Geometry: final body of the model. Coordinates: model frame, mm. A direction names the side the tool comes from. Give positions to 0.01 mm unless a question says otherwise; leave off trailing zeros. Loops run counter-clockwise (first coordinate to the right, second up) from the corner with the lowest first, then second, coordinate; pieces in that order, holes last. Notation, with made-up numbers: (-8, 59) - (20, 59) arc R20 cw to (20, 76) - close; hole circle Ø1 at (29, 48). An arc over 180 degrees is marked (long way). Answer in a Markdown table with one row per item.
from build123d import *

# Parameters (mm, degrees)
SKETCH1_R           = 1.5
BOSS_EXTRUDE1_DEPTH = 38.15
SKETCH4_W           = 9.31
SKETCH4_H           = 38.15
CUT_EXTRUDE2_DEPTH  = 45


with BuildPart() as part:
    # Sketch1 → Boss-Extrude1 (new body)
    with BuildSketch(Plane(origin=(0, 0, 0), x_dir=(1, 0, 0), z_dir=(0, 1, 0))):
        with BuildLine():
            Line((-43.3, 25.002199903), (-19.589917361, 15.692199903))
            ThreePointArc((-19.589917361, 15.692199903), (25.1, 0), (-19.589917361, -15.692199903))
            Line((-19.589917361, -15.692199903), (-43.3, -25.002199903))
            ThreePointArc((-43.3, -25.002199903), (50, 0), (-43.3, 25.002199903))
        make_face()
        with Locations(Location((8, -35.55, 0), (0, 0, 270))):
            Circle(SKETCH1_R, mode=Mode.SUBTRACT)
        with Locations(Location((-8, -35.55, 0), (0, 0, 90))):
            Circle(SKETCH1_R, mode=Mode.SUBTRACT)
        with Locations(Location((8, 35.55, 0), (0, 0, 90))):
            Circle(SKETCH1_R, mode=Mode.SUBTRACT)
        with Locations(Location((-8, 35.55, 0), (0, 0, 270))):
            Circle(SKETCH1_R, mode=Mode.SUBTRACT)
        with Locations(Location((35.55, 8, 0), (0, 0, 270))):
            Circle(SKETCH1_R, mode=Mode.SUBTRACT)
        with Locations(Location((35.55, -8, 0), (0, 0, 90))):
            Circle(SKETCH1_R, mode=Mode.SUBTRACT)
    extrude(amount=BOSS_EXTRUDE1_DEPTH)

    # Sketch4 → Cut-Extrude2 (cut)
    with BuildSketch(Plane.ZY.offset(43.3)):
        with Locations((-20.347199903, 19.075)):
            Rectangle(SKETCH4_W, SKETCH4_H)
        with Locations((20.347199903, 19.075)):
            Rectangle(SKETCH4_W, SKETCH4_H)
    extrude(amount=-CUT_EXTRUDE2_DEPTH, mode=Mode.SUBTRACT)


solid = part.part
Q1. Cut plane C-C (x = 35.55). Output: boundary loops of the cut face in (y, z).
Check values:
| item | result |
|---|---|
| outline | (0, -35.16) - (38.15, -35.16) - (38.15, -9.5) - (0, -9.5) - close; (0, -6.5) - (38.15, -6.5) - (38.15, 6.5) - (0, 6.5) - close; (0, 9.5) - (38.15, 9.5) - (38.15, 35.16) - (0, 35.16) - close |
Q2. Cut plane A-A (x = 0). Output: boundary loops of the cut face in (y, z).
Check values:
| item | result |
|---|---|
| outline | (0, -50) - (38.15, -50) - (38.15, -25.1) - (0, -25.1) - close; (0, 25.1) - (38.15, 25.1) - (38.15, 50) - (0, 50) - close |
Q3. First-contact query: pin 1 (12 mm diameter, centred on x = -8.5, y = 23.5, fed in from +Z); pin 2 (4 mm diameter, centred on x = 26, y = 17, fed in from +Z); pin 3 (1.8 mm diameter, centred on x = 8, z = 35.55, fed in from -Y); pin 4 (3.5 mm diameter, centred on x = 8, z = -35.55, fed in from +Y). Flat tips, straight axial feed; report the tip coordinate or a pass-through.
Check values:
| item | result |
|---|---|
| pin 1 | z = 49.94 |
| pin 2 | z = 43.86 |
| pin 3 | through |
| pin 4 | y = 38.15 |
Q4. Reachability of faces 1 (the flat face through (-23, 19, -25.002)), 2 (the cylindrical face through (7.425, 18.808, 36.936)) from +Z, -Z, +X, -X, +Y, -Y: full face, straight path, thin tool, end or side. Return the list, or none.
Check values:
| item | result |
|---|---|
| face 1 | -X, +Y, -Y |
| face 2 | +Y, -Y |
Q5. Cut plane B-B (y = 15.5). Output: boundary loops of the cut face in (x, z).
Check values:
| item | result |
|---|---|
| outline | (-43.3, -25) arc R50 ccw (long way) to (-43.3, 25) - (-2.21, 25) arc R25.1 cw (long way) to (-2.21, -25) - close; hole circle Ø3 at (-8, -35.55); hole circle Ø3 at (-8, 35.55); hole circle Ø3 at (8, -35.55); hole circle Ø3 at (8, 35.55); hole circle Ø3 at (35.55, -8); hole circle Ø3 at (35.55, 8) |
Q6. Material intervals for line 1 along X through (y, z) = (25, -35); line 2 along X through (y, z) = (19.5, 0), sorted ascending.
Check values:
| item | result |
|---|---|
| line 1 | -35.71 to -9.4, -6.6 to 6.6, 9.4 to 35.71 |
| line 2 | 25.1 to 50 |
Q7. Draft query along Z for faces 3 (the cylindrical face through (34.063, 18.808, 8.195)), 4 (the cylindrical face through (25.093, 18.808, -0.583)), 5 (the cylindrical face through (49.966, 18.808, 1.832)), 6 (the flat face through (23.4, 0, 10.4)). Return one class per face: pulls with the +Z half, pulls with the -Z half, needs draft (parallel to the pull), parting line crosses it, or undercut.
Check values:
| item | result |
|---|---|
| face 3 | undercut |
| face 4 | undercut |
| face 5 | parting line crosses it |
| face 6 | needs draft |
Q8. Cut plane D-D (z = -35.55). Output: boundary loops of the cut face in (x, y), and give its area (3 significant figures).
Check values:
| item | result |
|---|---|
| outline | (-35.16, 0) - (-9.5, 0) - (-9.5, 38.15) - (-35.16, 38.15) - close; (-6.5, 0) - (6.5, 0) - (6.5, 38.15) - (-6.5, 38.15) - close; (9.5, 0) - (35.16, 0) - (35.16, 38.15) - (9.5, 38.15) - close |
| area | 2,450 mm² |
